```python
from build123d import *

# Parameters (mm, degrees)
SKETCH1_W           = 40
SKETCH1_H           = 200
SKETCH1_R           = 2.5
BOSS_EXTRUDE1_DEPTH = 5


with BuildPart() as part:
    # Sketch1 → Boss-Extrude1 (new body)
    with BuildSketch(Plane.XY):
        with Locations((-20, -100)):
            Rectangle(SKETCH1_W, SKETCH1_H)
        with Locations((-20, -185)):
            Circle(SKETCH1_R, mode=Mode.SUBTRACT)
        with BuildLine():
            Line((-17, -107.376368338), (-17, -157.376368338))
            ThreePointArc((-17, -157.376368338), (-20, -160.376368338), (-23, -157.376368338))
            Line((-23, -157.376368338), (-23, -107.376368338))
            ThreePointArc((-23, -107.376368338), (-20, -104.376368338), (-17, -107.376368338))
        make_face(mode=Mode.SUBTRACT)
    extrude(amount=BOSS_EXTRUDE1_DEPTH)


solid = part.part
```
Input: part model. Units: mm. Frame: model coordinates. A direction names the side the tool comes from. Coordinates: 2 decimals unless noted, no trailing zeros. Order: outer loops, then holes, each group sorted by start corner. A loop starts at its lowest first (then second) coordinate and runs counter-clockwise, first axis right, second up. Notation, with made-up numbers: (81.25, 0.25) - (88.25, 0.25) arc R23 ccw to (88.25, 9.25) - close; hole circle Ø7 at (-3.75, 33.25). An arc over 180 degrees is marked (long way). Put each result on its own line as item: value.
1. Cut plane D-D on y = -185. Return the cut outline in (x, z).
Report:
outline: (-40, 0) - (-22.5, 0) - (-22.5, 5) - (-40, 5) - close; (-17.5, 0) - (0, 0) - (0, 5) - (-17.5, 5) - close
2. Draft query along X for faces 1 (the face through (-20, -99, 5)), 2 (the face through (-23, -133, 2)), 3 (the face through (0, -101, 2)). Return one class per face: pulls with the +X half, pulls with the -X half, needs draft (parallel to the pull), parting line crosses it, or undercut.
Report:
face 1: needs draft
face 2: undercut
face 3: pulls with the +X half
3. Cut plane B-B on z = 1.2. Return the cut outline in (x, y).
Report:
outline: (-40, -200) - (0, -200) - (0, 0) - (-40, 0) - close; hole (-23, -157.38) arc R3 ccw to (-17, -157.38) - (-17, -107.38) arc R3 ccw to (-23, -107.38) - close; hole circle Ø5 at (-20, -185)
4. Cut plane A-A on y = -138. Return the cut outline in (x, z).
Report:
outline: (-40, 0) - (-23, 0) - (-23, 5) - (-40, 5) - close; (-17, 0) - (0, 0) - (0, 5) - (-17, 5) - close
5. Line query: line 1 along Y through (x, z) = (-20, 2.8); line 2 along X through (y, z) = (-157.5, 1.35); line 3 along X through (y, z) = (-185, 2.75). Output: solid intervals per line, ascending.
Report:
line 1: y = -200 to -187.5, -182.5 to -160.38, -104.38 to 0
line 2: x = -40 to -23, -17 to 0
line 3: x = -40 to -22.5, -17.5 to 0
6. Reachability of faces 4 (the face through (-20, -200, 2)), 5 (the face through (-19.934, -160.376, 2.465)) from +Z, -Z, +X, -X, +Y, -Y: full face, straight path, thin tool, end or side. Return the list, or none.
Report:
face 4: +Z, -Z, +X, -X, -Y
face 5: +Z, -Z
7. Cut plane C-C on x = -20. Return the cut outline in (y, z), then the cut area to 3 significant figures.
Report:
outline: (-200, 0) - (-187.5, 0) - (-187.5, 5) - (-200, 5) - close; (-182.5, 0) - (-160.38, 0) - (-160.38, 5) - (-182.5, 5) - close; (-104.38, 0) - (0, 0) - (0, 5) - (-104.38, 5) - close
area: 695 mm2
